Build history of the part. All positions in model axes, mm. Face numbers are marked on the shaded views. A direction names the side the tool comes from. Coordinates: 2 decimals unless noted, no trailing zeros. Order: outer loops, then holes, each group sorted by start corner. A loop starts at its lowest first (then second) coordinate and runs counter-clockwise, first axis right, second up. Notation, with made-up numbers: (56.25, -11) - (77.25, -11) arc R18 cw to (77.25, 12) - close; hole circle Ø1 at (51, 84.25). An arc over 180 degrees is marked (long way). Return JSON: item names as keys, results as strings.
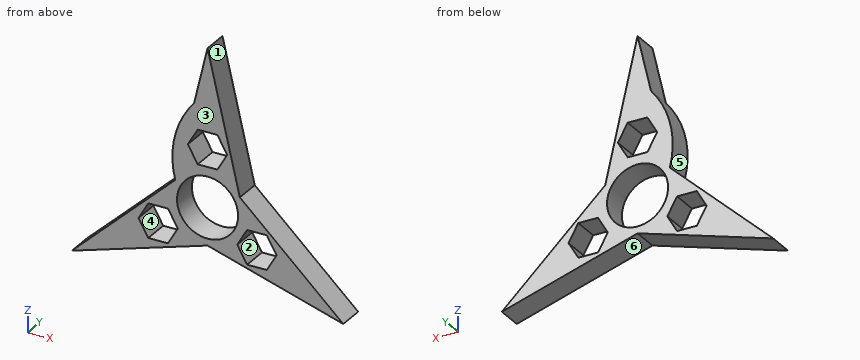
from build123d import *

# Parameters (mm, degrees)
F0_R     = 9.4
F1_DEPTH = 8
F2_DEPTH = 8


# Not quite as in the source:
# - a feature names something its author has since deleted; it is built from what else it names


with BuildPart() as f1:
    # F0 (on Front) → F1 (new body)
    with BuildSketch(Plane.XZ):
        Polygon((-4.1513990878, 30.4938093078), (-9.9419574161, 5.7399917905), (-41.7774577923, -24.1202265024), (0, -11.4799835809), (41.7774577923, -24.1202265024), (9.9419574161, 5.7399917905), (0, 48.2404530048), align=None)
        Polygon((-12.1738227533, -14.0285603702), (-18.2360010358, -14.0285603702), (-21.267090177, -8.7785599753), (-18.2360010358, -3.5285595804), (-12.1738227533, -3.5285595804), (-9.1427336121, -8.7785599753), align=None, mode=Mode.SUBTRACT)
        Polygon((18.2360010358, -3.5285595804), (21.267090177, -8.7785599753), (18.2360010358, -14.0285603702), (12.1738227533, -14.0285603702), (9.1427336121, -8.7785599753), (12.1738227533, -3.5285595804), align=None, mode=Mode.SUBTRACT)
        Circle(F0_R, mode=Mode.SUBTRACT)
        Polygon((6.0621782825, 17.5571199507), (3.0310891412, 12.3071195558), (-3.0310891412, 12.3071195558), (-6.0621782825, 17.5571199507), (-3.0310891412, 22.8071203455), (3.0310891412, 22.8071203455), align=None, mode=Mode.SUBTRACT)
    extrude(amount=F1_DEPTH)

    # F0 (on Front) → F2 (join)
    with BuildSketch(Plane.XZ):
        with BuildLine():
            ThreePointArc((-4.1513990878, 30.4938093078), (-10.107126805, 18.8328186432), (-9.9419574161, 5.7399917905))
            Line((-9.9419574161, 5.7399917905), (-4.1513990878, 30.4938093078))
        make_face()
        Polygon((-4.1513990878, 30.4938093078), (-9.9419574161, 5.7399917905), (-41.7774577923, -24.1202265024), (0, -11.4799835809), (41.7774577923, -24.1202265024), (9.9419574161, 5.7399917905), (0, 48.2404530048), align=None)
        Polygon((-12.1738227533, -14.0285603702), (-18.2360010358, -14.0285603702), (-21.267090177, -8.7785599753), (-18.2360010358, -3.5285595804), (-12.1738227533, -3.5285595804), (-9.1427336121, -8.7785599753), align=None, mode=Mode.SUBTRACT)
        Polygon((18.2360010358, -3.5285595804), (21.267090177, -8.7785599753), (18.2360010358, -14.0285603702), (12.1738227533, -14.0285603702), (9.1427336121, -8.7785599753), (12.1738227533, -3.5285595804), align=None, mode=Mode.SUBTRACT)
        Circle(F0_R, mode=Mode.SUBTRACT)
        Polygon((6.0621782825, 17.5571199507), (3.0310891412, 12.3071195558), (-3.0310891412, 12.3071195558), (-6.0621782825, 17.5571199507), (-3.0310891412, 22.8071203455), (3.0310891412, 22.8071203455), align=None, mode=Mode.SUBTRACT)
    extrude(amount=F2_DEPTH)


solid = f1.part
1. Cut at C-C on x = 5. Give the cut face in (y, z), plus the area to 3 significant figures.
Check values:
{"outline": "(-8, -12.99) - (0, -12.99) - (0, -7.96) - (-8, -7.96) - close; (-8, 7.96) - (0, 7.96) - (0, 15.72) - (-8, 15.72) - close; (-8, 19.4) - (0, 19.4) - (0, 26.87) - (-8, 26.87) - close", "area": "162 mm²"}
2. Cut at D-D on x = 19.5. Give the cut face in (y, z) (3 decimals).
Check values:
{"outline": "(-8, -17.38) - (0, -17.38) - (0, -11.839) - (-8, -11.839) - close; (-8, -5.718) - (0, -5.718) - (0, -3.225) - (-8, -3.225) - close"}
3. Mould opens along Z. For the marked faces 1, 2 and 3 say: pulls with the +Z half, pulls with the -Z half, needs draft (parallel to the pull), parting line crosses it, or undercut.
Check values:
{"face 1": "pulls with the +Z half", "face 2": "undercut", "face 3": "needs draft"}
4. Probe L1, parallel to Z at x = -4.5, y = -1.75; L2, parallel to X at y = -3, z = -6; L3, parallel to Z at x = 16, y = -4.5. List the from-to ranges inside material, lowest first.
Check values:
{"L1": "-12.84 to -8.25, 8.25 to 14.85, 20.26 to 30.08", "L2": "-22.46 to -19.66, -10.75 to -7.24, 7.24 to 10.75, 19.66 to 22.46", "L3": "-16.32 to -14.03, -3.53 to 0.06"}
5. Drop flat-ended pins along their axis: pin 1 (4 mm diameter, centred on x = 12.5, y = -2, fed in from +Z); pin 2 (6 mm diameter, centred on x = -3.5, z = -8.5, fed in from +Y); pin 3 (10 mm diameter, centred on x = -14.5, z = 30, fed in from -Y); pin 4 (3 mm diameter, centred on x = 26.5, y = -2.5, fed in from +Z). Give the stop position or say it passes through.
Check values:
{"pin 1": "z = 5.22", "pin 2": "y = 0", "pin 3": "through", "pin 4": "z = -8.38"}
6. Cut at A-A on y = -6. Give the cut face in (x, z), plus the area to 3 significant figures.
Check values:
{"outline": "(-41.78, -24.12) - (0, -11.48) - (41.78, -24.12) - (9.94, 5.74) - (0, 48.24) - (-4.15, 30.49) arc R27.27 ccw to (-9.94, 5.74) - close; hole (-21.27, -8.78) - (-18.24, -14.03) - (-12.17, -14.03) - (-9.14, -8.78) - (-12.17, -3.53) - (-18.24, -3.53) - close; hole circle Ø18.8 at (0, 0); hole (-6.06, 17.56) - (-3.03, 12.31) - (3.03, 12.31) - (6.06, 17.56) - (3.03, 22.81) - (-3.03, 22.81) - close; hole (9.14, -8.78) - (12.17, -14.03) - (18.24, -14.03) - (21.27, -8.78) - (18.24, -3.53) - (12.17, -3.53) - close", "area": "929 mm²"}
7. Tool access for the marked faces 4, 5 and 6: list every direction of +Z, -Z, +X, -X, +Y, -Y with a clear straight run to the whole face (end or side of a thin tool).
Check values:
{"face 4": "+Y, -Y", "face 5": "-X, +Y, -Y", "face 6": "-Z, +Y, -Y"}
8. Cut at B-B on z = -18. Give the cut face in (x, y).
Check values:
{"outline": "(-35.25, -8) - (-21.55, -8) - (-21.55, 0) - (-35.25, 0) - close; (21.55, -8) - (35.25, -8) - (35.25, 0) - (21.55, 0) - close"}
